Geometry: final body of the model. Coordinates: model frame, mm. A direction names the side the tool comes from. Coordinates: 2 decimals unless noted, no trailing zeros. Order: outer loops, then holes, each group sorted by start corner. A loop starts at its lowest first (then second) coordinate and runs counter-clockwise, first axis right, second up. Notation, with made-up numbers: (-17, -39.5) - (-6, -39.5) arc R15 ccw to (-6, -21.5) - close; hole circle Ø10 at (52, 47.25). An arc over 180 degrees is marked (long way). Use one line per item in the form item = value. Start each with the question number.
```python
from build123d import *

# Parameters (mm, degrees)
SKETCH1_R           = 4.7625
BOSS_EXTRUDE1_DEPTH = 3.175
SKETCH2_W           = 6.35
SKETCH2_H           = 3.175
SKETCH2_W_2         = 6.2738
CUT_EXTRUDE1_DEPTH  = 3.175


with BuildPart() as part:
    # Sketch1 → Boss-Extrude1 (new body)
    with BuildSketch(Plane.XY):
        with BuildLine():
            Line((7.987675642, 20.35683), (7.987675642, 0))
            Line((7.987675642, 0), (27.037675642, 0))
            Line((27.037675642, 0), (27.037675642, 9.358307372))
            ThreePointArc((27.037675642, 9.358307372), (27.037675642, 31.355352628), (7.987675642, 20.35683))
        make_face()
        with Locations((20.687675642, 20.35683)):
            Circle(SKETCH1_R, mode=Mode.SUBTRACT)
    extrude(amount=BOSS_EXTRUDE1_DEPTH)

    # Sketch2 → Cut-Extrude1 (cut)
    with BuildSketch(Plane.XZ):
        with Locations((11.162675642, 1.5875)):
            Rectangle(SKETCH2_W, SKETCH2_H)
        with Locations((23.900775642, 1.5875)):
            Rectangle(SKETCH2_W_2, SKETCH2_H)
    extrude(amount=-CUT_EXTRUDE1_DEPTH, mode=Mode.SUBTRACT)


solid = part.part
```
(1) Cut plane C-C on y = 21. Return the cut outline in (x, z) (3 decimals).
(2) Cut plane B-B on x = 19. Return the cut outline in (y, z) (3 decimals), plus the area to 3 significant figures.
(3) Set-up query: faces 1 (the flat face through (21, 13, 3.175)), 2 (the flat face through (11, 3.175, 2)), 3 (the flat face through (20.764, 2, 2)). Return all of +Z, -Z, +X, -X, +Y, -Y with unobstructed straight access to the full face (end or side cutting, diameter ignored); none if empty.
(4) Cut plane D-D on y = 5. Return the cut outline in (x, z) (3 decimals).
(5) Draft query along Y for faces 4 (the flat face through (7.988, 12, 2)), 5 (the cylindrical face through (23.25, 24.37, 1.57)), 6 (the flat face through (24, 3.175, 2)). Return one class per face: released by +Y, released by -Y, zero draft, split by the parting line, or undercut.
(6) Cut plane A-A on z = 2.2. Return the cut outline in (x, y) (1 decimal).
(7) Material intervals for L1, parallel to X at y = 3.5, z = 1.25; L2, parallel to Y at x = 24.5, z = 0.75 (3 decimals); L3, parallel to Y at x = 17, z = 1.6, sorted ascending. Write a range as from..to.
(8) Contact query for flat-ended pins moving along their axis: pin 1 Ø1.6 at (y, z) = (1.5, 2) entering from -X; pin 2 Ø1 at (x, z) = (13, 0.5) entering from -Y (3 decimals); pin 3 Ø1 at (y, z) = (18, 1.5) entering from +X. Output: stop coordinate, or through.
Check sheet entries:
q1.outline = (8.004, 0) - (15.969, 0) - (15.969, 3.175) - (8.004, 3.175) - close; (25.407, 0) - (33.371, 0) - (33.371, 3.175) - (25.407, 3.175) - close
q2.outline = (0, 0) - (15.903, 0) - (15.903, 3.175) - (0, 3.175) - close; (24.81, 0) - (32.944, 0) - (32.944, 3.175) - (24.81, 3.175) - close
q2.area = 76.3 mm^2
q3.face_1 = +Z, +X, -X, +Y, -Y
q3.face_2 = +Z, -Z, -X, -Y
q3.face_3 = +Z, -Z, +X, -Y
q4.outline = (7.988, 0) - (27.038, 0) - (27.038, 3.175) - (7.988, 3.175) - close
q5.face_4 = zero draft
q5.face_5 = undercut
q5.face_6 = released by -Y
q6.outline = (8, 3.2) - (14.3, 3.2) - (14.3, 0) - (20.8, 0) - (20.8, 3.2) - (27, 3.2) - (27, 9.4) arc R12.7 ccw (long way) to (8, 20.4) - close; hole circle Ø9.5 at (20.7, 20.4)
q7.L1 = 7.99..27.04
q7.L2 = 3.175..17.502, 23.211..32.471
q7.L3 = 0..17.34, 23.37..32.51
q8.pin_1 = 14.34
q8.pin_2 = 3.175
q8.pin_3 = 33.25
